from build123d import *

# Parameters (mm, degrees)
BOSS_EXTRUDE1_DEPTH     = 11.90625
SKETCH2_W               = 12.7
SKETCH2_H               = 38.149612403
SKETCH2_W_2             = 38.149612403
SKETCH2_H_2             = 12.7
CUT_EXTRUDE1_DEPTH      = 683.603309975
F_1_4_CLEARANCE_HOLE1_D = 6.7564
SKETCH8_W               = 482.6
SKETCH8_H               = 482.6
CUT_EXTRUDE4_DEPTH      = 683.603309975
SKETCH12_W              = 6.35
SKETCH12_H              = 76.249612403
SKETCH12_W_2            = 76.249612403
SKETCH12_H_2            = 6.35
CUT_EXTRUDE6_DEPTH      = 683.603309975


with BuildPart() as part:
    # Sketch1 → Boss-Extrude1 (new body)
    with BuildSketch(Plane(origin=(0, 0, 0), x_dir=(1, 0, 0), z_dir=(0, 1, 0))):
        with BuildLine():
            Line((-406.4, 0), (-482.6, 0))
            ThreePointArc((-482.6, 0), (0, 482.6), (482.6, 0))
            Line((482.6, 0), (406.4, 0))
            ThreePointArc((406.4, 0), (0, 406.4), (-406.4, 0))
        make_face()
    extrude(amount=BOSS_EXTRUDE1_DEPTH)

    # Sketch2 → Cut-Extrude1 (cut, through all)
    with BuildSketch(Plane(origin=(0, 11.90625, 0), x_dir=(1, 0, 0), z_dir=(0, 1, 0))):
        with Locations((0, 425.425193799)):
            Rectangle(SKETCH2_W, SKETCH2_H)
        with Locations((425.425193799, 0)):
            Rectangle(SKETCH2_W_2, SKETCH2_H_2)
        with Locations((0, -425.425193799)):
            Rectangle(SKETCH2_W, SKETCH2_H)
        with Locations((-425.425193799, 0)):
            Rectangle(SKETCH2_W_2, SKETCH2_H_2)
    extrude(amount=-CUT_EXTRUDE1_DEPTH, mode=Mode.SUBTRACT)

    # 1/4 Clearance Hole1 (through all)
    with Locations(Plane(origin=(0, 11.90625, 0), x_dir=(1, 0, 0), z_dir=(0, 1, 0))):
        with Locations((-365.700877383, 211.1375), (-31.75, 419.1), (-31.75, 450.85), (-419.1, 31.75), (-450.85, 31.75), (-211.1375, 365.700877383)):
            Hole(F_1_4_CLEARANCE_HOLE1_D / 2)

    # Sketch8 → Cut-Extrude4 (cut, through all)
    with BuildSketch(Plane(origin=(0, 11.90625, 0), x_dir=(1, 0, 0), z_dir=(0, 1, 0))):
        with Locations((241.3, 241.3)):
            Rectangle(SKETCH8_W, SKETCH8_H)
    extrude(amount=-CUT_EXTRUDE4_DEPTH, mode=Mode.SUBTRACT)

    # Sketch12 → Cut-Extrude6 (cut, through all)
    with BuildSketch(Plane(origin=(0, 11.90625, 0), x_dir=(1, 0, 0), z_dir=(0, 1, 0))):
        with Locations((-3.175, 444.475193799)):
            Rectangle(SKETCH12_W, SKETCH12_H)
        with Locations((-444.475193799, 3.175)):
            Rectangle(SKETCH12_W_2, SKETCH12_H_2)
    extrude(amount=-CUT_EXTRUDE6_DEPTH, mode=Mode.SUBTRACT)


solid = part.part
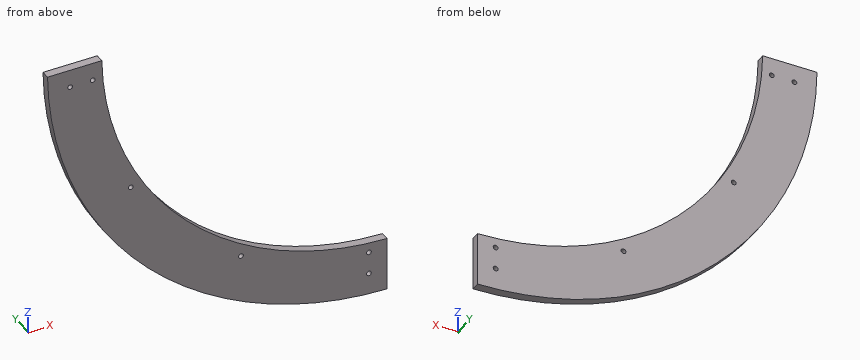
Work out the finished part from the listing and answer in its coordinate system (mm). Coordinates: 2 decimals unless noted, no trailing zeros. Loops run counter-clockwise (first coordinate to the right, second up) from the corner with the lowest first, then second, coordinate; pieces in that order, holes last. Notation, with made-up numbers: M -20,12.5 L 16,12.5 A14 cw 16,34.5 Z; hole C 36.5,33 d9. An arc over 180 degrees is marked long. Answer in a Markdown table with one row per item. Add a question column.
1. Find section A-A, the plane y = 9.5. Write down the section's boundary in (x, z), then the cut area to 3 significant figures.
2. Find section B-B, the plane x = -284.5. Write down the section's boundary in (y, z), then the cut area to 3 significant figures.
3. Flat-ended cylindrical pins translate along their axes: P1, Ø4, axis at y = 1.5, z = -343.5, coming from the -X side; P2, Ø1, axis at y = 10, z = -252, coming from the +X side; P3, Ø1.5, axis at x = -79.5, y = 2, coming from the -Z side; P4, Ø8, axis at x = -351, z = -190.5, coming from the -Y side. Find the tip coordinate at first contact, or state that the pin passes through.
4. Consider L1, parallel to Z at x = -31.75, y = 5.75; L2, parallel to X at y = 9.75, z = -29. Determine where each line is inside the solid, lowest interval first.
5. Find section C-C, the plane z = -255. Write down the section's boundary in (x, y), then the cut area to 3 significant figures.
Reported:
| question | item | result |
|---|---|---|
| 1 | outline | M -482.56,-6.35 A482.6 ccw -6.35,-482.56 L -6.35,-406.35 A406.4 cw -406.35,-6.35 Z; hole C -450.85,-31.75 d6.76; hole C -419.1,-31.75 d6.76; hole C -365.7,-211.14 d6.76; hole C -211.14,-365.7 d6.76; hole C -31.75,-450.85 d6.76; hole C -31.75,-419.1 d6.76 |
| 1 | area | 52,000 mm^2 |
| 2 | outline | M 0,-389.82 L 11.91,-389.82 L 11.91,-290.21 L 0,-290.21 Z |
| 2 | area | 1,190 mm^2 |
| 3 | P1 | stops at x = -341 |
| 3 | P2 | stops at x = -318.44 |
| 3 | P3 | stops at z = -476.13 |
| 3 | P4 | passes through |
| 4 | L1 | z = -481.55 to -454.23, -447.47 to -422.48, -415.72 to -405.16 |
| 4 | L2 | x = -481.73 to -452.81, -448.89 to -421.06, -417.14 to -405.36 |
| 5 | outline | M -409.73,0 L -316.44,0 L -316.44,11.91 L -409.73,11.91 Z |
| 5 | area | 1,110 mm^2 |
